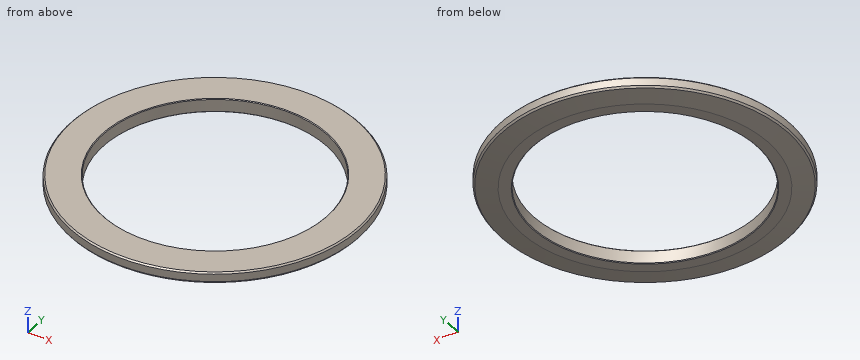
```python
from build123d import *
from OCP.BRepFilletAPI import BRepFilletAPI_MakeChamfer

# Parameters (mm, degrees)
SKETCH_1_R      = 20.575
SKETCH_1_R_2    = 15.9
EXTRUDE_1_DEPTH = 1.92
CHAMFER_1_SIZE  = 3
CHAMFER_1_SIZE2 = 0.4
CHAMFER_2_SIZE  = 0.2
CHAMFER_2_SIZE2 = 0.232811476
CHAMFER_3_SIZE  = 0.1


with BuildPart() as part:
    # Эскиз1 → Бобышка-Вытянуть1 (new body)
    with BuildSketch(Plane.XY):
        Circle(SKETCH_1_R)
        Circle(SKETCH_1_R_2, mode=Mode.SUBTRACT)
    extrude(amount=EXTRUDE_1_DEPTH)

    # Фаска1
    chamfer_1_edges = [part.edges().sort_by_distance(p)[0] for p in [
        (-20.575, 0, 0),
    ]]
    chamfer_1_side = [part.faces().sort_by_distance(p)[0] for p in [
        (-19.993051119, 0, 0),
    ]]
    chamfer(chamfer_1_edges, length=CHAMFER_1_SIZE, length2=CHAMFER_1_SIZE2, reference=chamfer_1_side[0])

    # Фаска2: one chamfer whose edges measure the first distance from different faces: ONE call of the kernel's chamfer builder (chamfer() names one face for all edges)
    chamfer_2_edges_1 = [part.edges().sort_by_distance(p)[0] for p in [
        (-20.575, 0, 1.92),
    ]]
    chamfer_2_edges_2 = [part.edges().sort_by_distance(p)[0] for p in [
        (-20.575, 0, 0.4),
    ]]
    chamfer_2_side_2 = [part.faces().sort_by_distance(p)[0] for p in [
        (-19.075, 0, 0.2),
    ]]
    chamfer_2 = BRepFilletAPI_MakeChamfer(part.part.solid().wrapped)
    for e in chamfer_2_edges_1:
        chamfer_2.Add(CHAMFER_2_SIZE, e.wrapped)
    for e in chamfer_2_edges_2:
        chamfer_2.Add(CHAMFER_2_SIZE, CHAMFER_2_SIZE2, e.wrapped, chamfer_2_side_2[0].wrapped)  # the first distance lies on this face
    add(Compound.cast(chamfer_2.Shape()), mode=Mode.REPLACE)

    # Фаска3
    chamfer_3_edges = [part.edges().sort_by_distance(p)[0] for p in [
        (-15.9, 0, 0),
        (-15.9, 0, 1.92),
    ]]
    chamfer(chamfer_3_edges, length=CHAMFER_3_SIZE)


solid = part.part
```
Geometry: final body of the model. Coordinates: model frame, mm. Round coordinates to 2 decimals unless told otherwise and drop trailing zeros. Order: outer loops, then holes, each group sorted by start corner. A loop starts at its lowest first (then second) coordinate and runs counter-clockwise, first axis right, second up. Notation, with made-up numbers: (87.5, -21.5) -> (105.5, -21.5) arc R9 cw to (105.5, -8.5) -> close; hole circle Ø9 at (15.25, 11.5). An arc over 180 degrees is marked (long way). Write each question's results on one line, items separated by ' | '.
Q1. Ray query, line 1 along Y through (x, z) = (0, 1.1) (3 decimals); line 2 along X through (y, z) = (-3.5, 0.4); line 3 along Y through (x, z) = (2.5, 1.4). Return the intervals inside material, ascending.
Response values:
line 1: -20.575 to -15.9, 15.9 to 20.575 | line 2: -20.09 to -15.51, 15.51 to 20.09 | line 3: -20.42 to -15.7, 15.7 to 20.42
Q2. Pin query (flat end, axial travel): pin 1 Ø1 at (y, z) = (-15, 0.5) entering from +X. Return the tip coordinate at first contact, or that it passes through.
Response values:
pin 1: x = 14.58
Q3. Section query A-A (z = 1). Output: boundary loops of the cut face in (x, y) (3 decimals).
Response values:
outline: circle Ø41.15 at (0, 0); hole circle Ø31.8 at (0, 0)
